Can you work these out from the model? Positions are in its coordinate system, mm. A direction names the side the tool comes from. Round coordinates to 2 decimals unless told otherwise and drop trailing zeros. Order: outer loops, then holes, each group sorted by start corner. A loop starts at its lowest first (then second) coordinate and runs counter-clockwise, first axis right, second up. Notation, with made-up numbers: M 62.25,-4.75 L 111.25,-4.75 A15 cw 111.25,5.25 Z; hole C -15.5,9 d8. An arc over 180 degrees is marked long. Answer as a JSON object with one key per item and string values. Group by question number.
```python
from build123d import *

# Parameters (mm, degrees)
SKETCH1_W           = 31
SKETCH1_H           = 22.5
BOSS_EXTRUDE1_DEPTH = 7.5
SKETCH2_W           = 15
SKETCH2_H           = 4.5
BOSS_EXTRUDE2_DEPTH = 2.5
SKETCH3_R           = 0.5
BOSS_EXTRUDE3_DEPTH = 7


with BuildPart() as part:
    # Sketch1 → Boss-Extrude1 (new body)
    with BuildSketch(Plane(origin=(0, 0, 0), x_dir=(1, 0, 0), z_dir=(0, 1, 0))):
        Rectangle(SKETCH1_W, SKETCH1_H)
    extrude(amount=BOSS_EXTRUDE1_DEPTH)

    # Sketch2 → Boss-Extrude2 (add)
    with BuildSketch(Plane.ZY.offset(15.5)):
        with Locations((3.75, 5.25)):
            Rectangle(SKETCH2_W, SKETCH2_H)
    extrude(amount=BOSS_EXTRUDE2_DEPTH)

    # Sketch3 → Boss-Extrude3 (add)
    with BuildSketch(Plane.ZY.offset(18)):
        with Locations(Location((-2.45, 6.2, 0), (0, 0, 180))):
            Circle(SKETCH3_R)
        with Locations(Location((0.05, 6.2, 0), (0, 0, 180))):
            Circle(SKETCH3_R)
        with Locations(Location((2.55, 6.2, 0), (0, 0, 180))):
            Circle(SKETCH3_R)
        with Locations(Location((5.05, 6.2, 0), (0, 0, 180))):
            Circle(SKETCH3_R)
        with Locations(Location((7.55, 6.2, 0), (0, 0, 180))):
            Circle(SKETCH3_R)
        with Locations(Location((10.05, 6.2, 0), (0, 0, 180))):
            Circle(SKETCH3_R)
        with Locations(Location((-2.45, 4.7, 0), (0, 0, 180))):
            Circle(SKETCH3_R)
        with Locations(Location((0.05, 4.7, 0), (0, 0, 180))):
            Circle(SKETCH3_R)
        with Locations(Location((2.55, 4.7, 0), (0, 0, 180))):
            Circle(SKETCH3_R)
        with Locations(Location((5.05, 4.7, 0), (0, 0, 180))):
            Circle(SKETCH3_R)
        with Locations(Location((7.55, 4.7, 0), (0, 0, 180))):
            Circle(SKETCH3_R)
        with Locations(Location((10.05, 4.7, 0), (0, 0, 180))):
            Circle(SKETCH3_R)
    extrude(amount=BOSS_EXTRUDE3_DEPTH)


solid = part.part
```
1) For pin 1 (0.8 mm diameter, centred on x = -16.5, y = 5.5, fed in from -Z); pin 2 (1.3 mm diameter, centred on y = 5.5, z = 4, fed in from -X), each with a flat end and sliding along its axis, tell me the tip position at first contact or that it passes through.
2) I need wall thicknesses on line 1 along Z through (x, y) = (-18.5, 5); line 2 along X through (y, z) = (5.75, -6.75); line 3 along X through (y, z) = (5.75, -1). Which ranges of each line are inside material? Lowest first, please.
3) If we section it at A-A on x = -20: Count the separate pieces of the cut face and the enclosed holes in it, plus the area to 3 significant figures.
4) If we section it at B-B on z = 7.55: Write out the boundary of the cut face in (x, y).
5) If we section it at C-C on y = 3.75: Write out the boundary of the cut face in (x, z).
6) We'd pull the mould along Y, two halves only. Please class faces 3 (the face through (-21.45, 6.5, 7.95)), 4 (the face through (-25, 4.7, -2.4)), 5 (the face through (-17, 3, 4)), 6 (the face through (-21.451, 4.892, 2.088)): +Y half, -Y half, draft (parallel to the pull), parting line (faces both ways), or undercut.
7) Which directions (+Z, -Z, +X, -X, +Y, -Y) give clear straight access to the entire face, cutting with the end or side of a thin tool? Please do faces 1 (the face through (-25, 5, 0)), 2 (the face through (-21.451, 5.188, -2.342)).
8) If we section it at D-D on z = -4.5: Write out the boundary of the cut face in (x, y), plus the area to 4 significant figures.
Findings:
{
 "1": {"pin 1": "stops at z = -3.75", "pin 2": "stops at x = -18"},
 "2": {"line 1": "z = -2.85 to -2.05, -0.35 to 0.45, 2.15 to 2.95, 4.65 to 5.45, 7.15 to 7.95, 9.65 to 10.45", "line 2": "x = -15.5 to 15.5", "line 3": "x = -18 to 15.5"},
 "3": {"separate pieces": "12", "enclosed holes": "0", "area": "9.42 mm^2"},
 "4": {"outline": "M -25,4.2 L -18,4.2 L -18,3 L -15.5,3 L -15.5,0 L 15.5,0 L 15.5,7.5 L -18,7.5 L -18,6.7 L -25,6.7 L -25,5.7 L -18,5.7 L -18,5.2 L -25,5.2 Z"},
 "5": {"outline": "M -18,-3.75 L -15.5,-3.75 L -15.5,-11.25 L 15.5,-11.25 L 15.5,11.25 L -18,11.25 Z"},
 "6": {"face 3": "undercut", "face 4": "draft", "face 5": "-Y half", "face 6": "undercut"},
 "7": {"face 1": "+Z, -Z, -X, +Y, -Y", "face 2": "-X"},
 "8": {"outline": "M -15.5,0 L 15.5,0 L 15.5,7.5 L -15.5,7.5 Z", "area": "232.5 mm^2"}
}
